Can you work these out from the model? Positions are in its coordinate system, mm. Face numbers are marked on the shaded views. A direction names the side the tool comes from. Give positions to 0.01 mm unless a question says otherwise; leave off trailing zeros. Loops run counter-clockwise (first coordinate to the right, second up) from the corner with the lowest first, then second, coordinate; pieces in that order, holes last. Notation, with made-up numbers: (20.25, -7.5) - (62.25, -7.5) arc R21 cw to (62.25, 23.5) - close; hole circle Ø7 at (51.5, 73). An arc over 180 degrees is marked (long way). Write item = value, one per line.
from build123d import *

# Parameters (mm, degrees)
SKETCH_1_R               = 44.5
EXTRUDE_1_DEPTH          = 42
HOLE_WIZARD_M4_1_D       = 3.3
HOLE_WIZARD_M4_1_DEPTH   = 12
HOLE_WIZARD_M4_1_TIP     = 0.991420021
SKETCH_4_R               = 2
CUT_EXTRUDE_1_DEPTH      = 10
PATTERN_CIRCULAR_1_COUNT = 4
SKETCH_5_W               = 19.478252765
SKETCH_5_H               = 48.547320344
CUT_EXTRUDE_2_DEPTH      = 10
SKETCH_6_W               = 5.245291094
SKETCH_6_H               = 29.052548629
CUT_EXTRUDE_3_DEPTH      = 10


with BuildPart() as part:
    # 草图1 → 凸台-拉伸1 (new body)
    with BuildSketch(Plane.XY):
        with Locations(Location((0, 0, 0), (0, 0, 180))):
            Circle(SKETCH_1_R)
    extrude(amount=EXTRUDE_1_DEPTH)

    # M4 螺纹孔的螺纹孔钻头1
    with Locations(Plane(origin=(15, 15, 0), x_dir=(-1, 0, 0), z_dir=(0, 0, -1))):
        with Locations((0, 0), (30, 0), (30, -30), (0, -30)):
            Hole(HOLE_WIZARD_M4_1_D / 2, depth=HOLE_WIZARD_M4_1_DEPTH)
            with Locations((0, 0, -(HOLE_WIZARD_M4_1_DEPTH + HOLE_WIZARD_M4_1_TIP / 2))):  # 118° drill point
                Cone(0, HOLE_WIZARD_M4_1_D / 2, HOLE_WIZARD_M4_1_TIP, mode=Mode.SUBTRACT)

    # 草图4 → 切除-拉伸1 (cut)
    with BuildSketch(Plane.XY.offset(42)):
        with Locations((0, 22)):
            Circle(SKETCH_4_R)
        with Locations((12.374368671, 12.374368671)):
            Circle(SKETCH_4_R)
    cut_extrude_1 = extrude(amount=-CUT_EXTRUDE_1_DEPTH, mode=Mode.SUBTRACT)

    # 阵列(圆周)1: 切除-拉伸1 ×4 about axis
    pattern_circular_1_axis = Axis((0, 0, 0), (0, 0, 1))
    for i in range(1, PATTERN_CIRCULAR_1_COUNT):
        add(cut_extrude_1.rotate(pattern_circular_1_axis, i * 360 / PATTERN_CIRCULAR_1_COUNT), mode=Mode.SUBTRACT)

    # 草图5 → 切除-拉伸2 (cut)
    with BuildSketch(Plane(origin=(0, 0, 0), x_dir=(-1, 0, 0), z_dir=(0, 0, -1))):
        with Locations((48.243799035, -1.742903496)):
            Rectangle(SKETCH_5_W, SKETCH_5_H)
    extrude(amount=-CUT_EXTRUDE_2_DEPTH, mode=Mode.SUBTRACT)

    # 草图6 → 切除-拉伸3 (cut)
    with BuildSketch(Plane.ZY.offset(38.504672652)):
        with Locations((5.335468617, -0.326949721)):
            Rectangle(SKETCH_6_W, SKETCH_6_H)
    extrude(amount=-CUT_EXTRUDE_3_DEPTH, mode=Mode.SUBTRACT)


solid = part.part
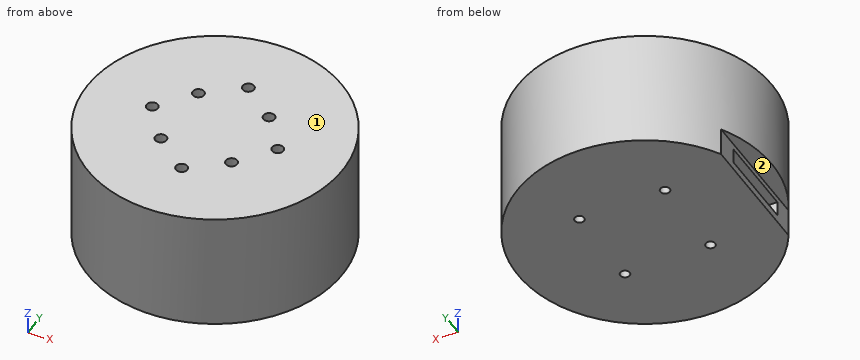
Q1. I need wall thicknesses on L1, parallel to Y at x = 0, z = 35; L2, parallel to X at y = -15, z = 9; L3, parallel to Z at x = 1.5, y = -22. Which ranges of each line are inside material? Lowest first, please.
Output:
L1 = -44.5 to -24, -20 to 20, 24 to 44.5
L2 = -38.5 to -16.65, -13.35 to 13.35, 16.65 to 41.9
L3 = 0 to 32
Q2. Imagine slicing it at A-A, the plane x = 22. Write out the boundary of the cut face in (y, z).
Output:
outline = (-38.68, 0) - (38.68, 0) - (38.68, 42) - (2, 42) - (2, 32) - (-2, 32) - (-2, 42) - (-38.68, 42) - close
Q3. Imagine slicing it at B-B, the plane z = 39.5. Give the number of separate pieces and of enclosed holes in the cut face, then the cut area to 3 significant figures.
Output:
separate_pieces = 1
enclosed_holes = 8
area = 6,120 mm2
Q4. For pin 1 (4.5 mm diameter, centred on x = 12.5, y = 12.5, fed in from +Z); pin 2 (10 mm diameter, centred on y = -34.5, z = 16.5, fed in from +X); pin 3 (3.5 mm diameter, centred on x = 0, y = 22, fed in from +Z); pin 4 (1 mm diameter, centred on y = 17.5, z = 5, fed in from -X), each with a flat end and sliding along its axis, tell me the tip position at first contact or that it passes through.
Output:
pin_1 = 42
pin_2 = 33.32
pin_3 = 32
pin_4 = -38.5
Q5. Which directions (+Z, -Z, +X, -X, +Y, -Y) give clear straight access to the entire face, cutting with the end or side of a thin tool? Please do the marked faces 1 and 2.
Output:
face_1 = +Z, +X, -X, +Y, -Y
face_2 = -Z, -X, +Y, -Y
Q6. Imagine slicing it at C-C, the plane z = 29. Write out the boundary of the cut face in (x, y), then the cut area to 3 significant figures.
Output:
outline = circle Ø89 at (0, 0)
area = 6,220 mm2
Q7. Imagine slicing it at D-D, the plane y = 5.5. Write out the boundary of the cut face in (x, z).
Output:
outline = (-44.16, 10) - (-38.5, 10) - (-38.5, 7.96) - (-28.5, 7.96) - (-28.5, 2.71) - (-38.5, 2.71) - (-38.5, 0) - (44.16, 0) - (44.16, 42) - (-44.16, 42) - close
